```python
from build123d import *

# Parameters (mm, degrees)
SKETCH1_R           = 3
BOSS_EXTRUDE1_DEPTH = 10
CHAMFER1_SIZE       = 1


with BuildPart() as part:
    # Sketch1 → Boss-Extrude1 (new body)
    with BuildSketch(Plane.XY):
        with BuildLine():
            Line((75.4, 25.4), (50, 25.4))
            Line((50, 25.4), (50, 47.8))
            ThreePointArc((50, 47.8), (49.121320344, 49.921320344), (47, 50.8))
            Line((47, 50.8), (-47, 50.8))
            ThreePointArc((-47, 50.8), (-49.121320344, 49.921320344), (-50, 47.8))
            Line((-50, 47.8), (-50, 25.4))
            Line((-50, 25.4), (-75.4, 25.4))
            Line((-75.4, 25.4), (-75.4, 47.8))
            ThreePointArc((-75.4, 47.8), (-76.278679656, 49.921320344), (-78.4, 50.8))
            Line((-78.4, 50.8), (-85.1, 50.8))
            ThreePointArc((-85.1, 50.8), (-87.221320344, 49.921320344), (-88.1, 47.8))
            Line((-88.1, 47.8), (-88.1, -22.4))
            ThreePointArc((-88.1, -22.4), (-87.221320344, -24.521320344), (-85.1, -25.4))
            Line((-85.1, -25.4), (85.1, -25.4))
            ThreePointArc((85.1, -25.4), (87.221320344, -24.521320344), (88.1, -22.4))
            Line((88.1, -22.4), (88.1, 47.8))
            ThreePointArc((88.1, 47.8), (87.221320344, 49.921320344), (85.1, 50.8))
            Line((85.1, 50.8), (78.4, 50.8))
            ThreePointArc((78.4, 50.8), (76.278679656, 49.921320344), (75.4, 47.8))
            Line((75.4, 47.8), (75.4, 25.4))
        make_face()
        with Locations((-19.05, 31.75)):
            Circle(SKETCH1_R, mode=Mode.SUBTRACT)
        with Locations((19.05, 31.75)):
            Circle(SKETCH1_R, mode=Mode.SUBTRACT)
        with Locations((19.05, -6.35)):
            Circle(SKETCH1_R, mode=Mode.SUBTRACT)
        with Locations((-19.05, -6.35)):
            Circle(SKETCH1_R, mode=Mode.SUBTRACT)
        with Locations((-81.75, 31.75)):
            Circle(SKETCH1_R, mode=Mode.SUBTRACT)
        with Locations((-81.75, -6.35)):
            Circle(SKETCH1_R, mode=Mode.SUBTRACT)
        with Locations(Location((81.75, -6.35, 0), (0, 0, 180))):
            Circle(SKETCH1_R, mode=Mode.SUBTRACT)
        with Locations(Location((81.75, 31.75, 0), (0, 0, 180))):
            Circle(SKETCH1_R, mode=Mode.SUBTRACT)
    extrude(amount=BOSS_EXTRUDE1_DEPTH)

    # Chamfer1
    chamfer1_edges = [part.edges().sort_by_distance(p)[0] for p in [
        (-81.75, 50.8, 10),
        (-87.221320344, 49.921320344, 10),
        (-62.7, 25.4, 0),
        (-50, 36.6, 0),
        (-49.121320344, 49.921320344, 0),
        (0, 50.8, 0),
        (-88.1, 12.7, 10),
        (49.121320344, 49.921320344, 0),
        (50, 36.6, 0),
        (62.7, 25.4, 0),
        (75.4, 36.6, 0),
        (76.278679656, 49.921320344, 0),
        (81.75, 50.8, 0),
        (87.221320344, 49.921320344, 0),
        (88.1, 12.7, 0),
        (87.221320344, -24.521320344, 0),
        (0, -25.4, 0),
        (-87.221320344, -24.521320344, 10),
        (-87.221320344, -24.521320344, 0),
        (-88.1, 12.7, 0),
        (-87.221320344, 49.921320344, 0),
        (-81.75, 50.8, 0),
        (-76.278679656, 49.921320344, 0),
        (-75.4, 36.6, 0),
        (0, -25.4, 10),
        (87.221320344, -24.521320344, 10),
        (88.1, 12.7, 10),
        (87.221320344, 49.921320344, 10),
        (81.75, 50.8, 10),
        (76.278679656, 49.921320344, 10),
        (-22.05, 31.75, 0),
        (-22.05, 31.75, 10),
        (-75.4, 36.6, 10),
        (75.4, 36.6, 10),
        (-84.75, 31.75, 0),
        (-84.75, 31.75, 10),
        (16.05, 31.75, 0),
        (62.7, 25.4, 10),
        (16.05, 31.75, 10),
        (16.05, -6.35, 0),
        (50, 36.6, 10),
        (16.05, -6.35, 10),
        (-22.05, -6.35, 0),
        (-22.05, -6.35, 10),
        (49.121320344, 49.921320344, 10),
        (-84.75, -6.35, 0),
        (-84.75, -6.35, 10),
        (0, 50.8, 10),
        (84.75, -6.35, 0),
        (84.75, -6.35, 10),
        (-49.121320344, 49.921320344, 10),
        (84.75, 31.75, 0),
        (84.75, 31.75, 10),
        (-50, 36.6, 10),
        (-62.7, 25.4, 10),
        (-76.278679656, 49.921320344, 10),
    ]]
    chamfer(chamfer1_edges, length=CHAMFER1_SIZE)


solid = part.part
```
Could you check a few things on this model? Use its own coordinates, in mm. A direction names the side the tool comes from. Round coordinates to 2 decimals unless told otherwise and drop trailing zeros. Loops run counter-clockwise (first coordinate to the right, second up) from the corner with the lowest first, then second, coordinate; pieces in that order, holes last. Notation, with made-up numbers: (64.25, 26) - (86.25, 26) arc R29 ccw to (86.25, 49) - close; hole circle Ø8 at (6, -4.5). An arc over 180 degrees is marked (long way). Answer in a Markdown table with one row per item. Add a question column.
(1) For faces 1 (the face through (48.703, 49.466, 9.618)), 2 (the face through (-76.697, 49.466, 0.382)), 3 (the face through (50, 36, 5)), which set-ups out of +Z, -Z, +X, -X, +Y, -Y let a thin tool reach every point of the face, with its end or its side?
(2) I'm going to push flat-ended pins straight in: pin 1 (3.5 mm diameter, centred on x = 81.75, y = -6.35, fed in from -Z) (3 decimals); pin 2 (7 mm diameter, centred on x = -19.05, y = -6.35, fed in from -Z). Where does each tip first touch, or does it pass through?
(3) I need wall thicknesses on line 1 along X through (y, z) = (44, 3.5); line 2 along Y through (x, z) = (-19.05, 7.75); line 3 along Y through (x, z) = (72.5, 5.25). Which ranges of each line are inside material? Lowest first, please.
(4) If we section it at B-B (x = 19.05): Please give me the cut outline in (y, z), plus the area to 3 significant figures.
(5) If we section it at A-A (z = 4.5): State how many separate pieces and enclosed holes the cut face has, plus the area to 3 significant figures.
(6) If we section it at C-C (x = -60): Please give me the cut outline in (y, z), plus the area to 3 significant figures.
Model answer:
| question | item | result |
|---|---|---|
| 1 | face 1 | +Z, +Y |
| 1 | face 2 | -Z, +Y |
| 1 | face 3 | +Z, -Z, +Y |
| 2 | pin 1 | passes through |
| 2 | pin 2 | stops at z = 0.5 |
| 3 | line 1 | x = -88.1 to -75.4, -50 to 50, 75.4 to 88.1 |
| 3 | line 2 | y = -25.4 to -9.35, -3.35 to 28.75, 34.75 to 50.8 |
| 3 | line 3 | y = -25.4 to 25.4 |
| 4 | outline | (-25.4, 1) - (-24.4, 0) - (-10.35, 0) - (-9.35, 1) - (-9.35, 9) - (-10.35, 10) - (-24.4, 10) - (-25.4, 9) - close; (-3.35, 1) - (-2.35, 0) - (27.75, 0) - (28.75, 1) - (28.75, 9) - (27.75, 10) - (-2.35, 10) - (-3.35, 9) - close; (34.75, 1) - (35.75, 0) - (49.8, 0) - (50.8, 1) - (50.8, 9) - (49.8, 10) - (35.75, 10) - (34.75, 9) - close |
| 4 | area | 636 mm² |
| 5 | separate pieces | 1 |
| 5 | enclosed holes | 8 |
| 5 | area | 11,900 mm² |
| 6 | outline | (-25.4, 1) - (-24.4, 0) - (24.4, 0) - (25.4, 1) - (25.4, 9) - (24.4, 10) - (-24.4, 10) - (-25.4, 9) - close |
| 6 | area | 506 mm² |
